Could you check a few things on this model? Use its own coordinates, in mm. A direction names the side the tool comes from. Round coordinates to 2 decimals unless told otherwise and drop trailing zeros. Loops run counter-clockwise (first coordinate to the right, second up) from the corner with the lowest first, then second, coordinate; pieces in that order, holes last. Notation, with made-up numbers: (2, 27) -> (25, 27) arc R19 cw to (25, 31) -> close; hole circle Ø9 at (75.5, 49.5). An arc over 180 degrees is marked (long way). One line per item, written item: value.
from build123d import *

# Parameters (mm, degrees)
SZKIC1_W                          = 25
SZKIC1_H                          = 22
SZKIC1_W_2                        = 21
SZKIC1_H_2                        = 18
WYCI_GNI_CIE_CIENKA_CIANKA1_DEPTH = 220
WYTNIJ_WYCI_GNI_CIE1_DEPTH        = 23
SZKIC3_R                          = 5
WYTNIJ_WYCI_GNI_CIE2_DEPTH        = 23
SZKIC4_R                          = 2
WYTNIJ_WYCI_GNI_CIE3_DEPTH        = 23


with BuildPart() as part:
    # Szkic1 → Wyciągnięcie-cienka ścianka1 (new body)
    with BuildSketch(Plane.XY):
        with Locations((12.5, -9.5)):
            Rectangle(SZKIC1_W, SZKIC1_H)
        with Locations((12.5, -9.5)):
            Rectangle(SZKIC1_W_2, SZKIC1_H_2, mode=Mode.SUBTRACT)
    extrude(amount=WYCI_GNI_CIE_CIENKA_CIANKA1_DEPTH)

    # Szkic2 → Wytnij-wyciągnięcie1 (cut, through all)
    with BuildSketch(Plane.XZ.offset(20.5)):
        with BuildLine():
            ThreePointArc((12.5, 0), (3.661165235, 3.661165235), (0, 12.5))
            Line((0, 12.5), (0, 0))
            Line((0, 0), (12.5, 0))
        make_face()
        with BuildLine():
            ThreePointArc((25, 12.5), (21.338834765, 3.661165235), (12.5, 0))
            Line((12.5, 0), (25, 0))
            Line((25, 0), (25, 12.5))
        make_face()
    extrude(amount=-WYTNIJ_WYCI_GNI_CIE1_DEPTH, mode=Mode.SUBTRACT)

    # Szkic3 → Wytnij-wyciągnięcie2 (cut, through all)
    with BuildSketch(Plane.XZ.offset(20.5)):
        with Locations((12.5, 12.5)):
            Circle(SZKIC3_R)
    extrude(amount=-WYTNIJ_WYCI_GNI_CIE2_DEPTH, mode=Mode.SUBTRACT)

    # Szkic4 → Wytnij-wyciągnięcie3 (cut, through all)
    with BuildSketch(Plane.XZ.offset(20.5)):
        with Locations((12.5, 60)):
            Circle(SZKIC4_R)
    extrude(amount=-WYTNIJ_WYCI_GNI_CIE3_DEPTH, mode=Mode.SUBTRACT)


solid = part.part
(1) If we section it at A-A, the plane z = 60: Please give me the cut outline in (x, y), then the cut area to 3 significant figures.
Recorded:
outline: (0, -20.5) -> (10.5, -20.5) -> (10.5, -18.5) -> (2, -18.5) -> (2, -0.5) -> (10.5, -0.5) -> (10.5, 1.5) -> (0, 1.5) -> close; (14.5, -20.5) -> (25, -20.5) -> (25, 1.5) -> (14.5, 1.5) -> (14.5, -0.5) -> (23, -0.5) -> (23, -18.5) -> (14.5, -18.5) -> close
area: 156 mm²
(2) For faces 5 (the face through (12, -0.5, 108)), 6 (the face through (12.24, 0.486, 61.983)), which set-ups out of +Z, -Z, +X, -X, +Y, -Y let a thin tool reach every point of the face, with its end or its side?
Recorded:
face 5: +Z, -Z
face 6: +Y, -Y
(3) If we section it at D-D, the plane z = 184: Please give me the cut outline in (x, y), then the cut area to 3 significant figures.
Recorded:
outline: (0, -20.5) -> (25, -20.5) -> (25, 1.5) -> (0, 1.5) -> close; hole (2, -18.5) -> (23, -18.5) -> (23, -0.5) -> (2, -0.5) -> close
area: 172 mm²
(4) Thinking about a two-plate mould opening in Y: for faces 1 (the face through (17.27, -19.51, 14)), 2 (the face through (23, -10, 111)), 3 (the face through (12, -18.5, 108)), 4 (the face through (12, 1.5, 108)), which applies, released by +Y, released by -Y, zero draft, split by the parting line, or undercut?
Recorded:
face 1: zero draft
face 2: undercut
face 3: undercut
face 4: released by +Y
(5) If we section it at B-B, the plane y = -9.5: Please give me the cut outline in (x, z).
Recorded:
outline: (0, 12.5) arc R12.5 ccw to (2, 5.72) -> (2, 220) -> (0, 220) -> close; (23, 5.72) arc R12.5 ccw to (25, 12.5) -> (25, 220) -> (23, 220) -> close
(6) If I drill on L1, parallel to Z at x = 12.5, y = 0; L2, parallel to X at y = -17.5, z = 123; L3, parallel to Y at x = 3, z = 211, over which ranges is the centre line in solid material (lowest first)?
Recorded:
L1: 0 to 7.5, 17.5 to 58, 62 to 220
L2: 0 to 2, 23 to 25
L3: -20.5 to -18.5, -0.5 to 1.5
(7) If we section it at C-C, the plane x = 4.25: Please give me the cut outline in (y, z).
Recorded:
outline: (-20.5, 3.11) -> (-18.5, 3.11) -> (-18.5, 220) -> (-20.5, 220) -> close; (-0.5, 3.11) -> (1.5, 3.11) -> (1.5, 220) -> (-0.5, 220) -> close
